Source: CAD feature listing. Evaluate the final solid. Frame: model axes, mm. A direction names the side the tool comes from. Round coordinates to 2 decimals unless told otherwise and drop trailing zeros. Loops run counter-clockwise (first coordinate to the right, second up) from the corner with the lowest first, then second, coordinate; pieces in that order, holes last. Notation, with made-up numbers: (62, 72) -> (71, 72) arc R31 ccw to (71, 111) -> close; hole circle Ø5 at (59, -21). An arc over 180 degrees is marked (long way). Put each result on its own line as item: value. Start each with the question number.
1. Material intervals for L1, parallel to Y at x = -5, z = 0; L2, parallel to Y at x = -9, z = -34; L3, parallel to Y at x = 22, z = -22.5, sorted ascending.
2. Cut plane A-A (x = -17). Return the cut outline in (y, z), then the cut area to 3 significant figures.
3. Cut plane B-B (y = -2). State how many separate pieces and enclosed holes the cut face has, then the cut area to 3 significant figures.
4. Set-up query: faces 4 (the flat face through (0, -22, 1)), 5 (the flat face through (17.426, 4, -1)), 6 (the flat face through (0, 5, 59)). Return all of +Z, -Z, +X, -X, +Y, -Y with unobstructed straight access to the full face (end or side cutting, diameter ignored); none if empty.
5. Contact query for flat-ended pins moving along their axis: pin 1 (1.2 mm diameter, centred on x = -24, z = -4, fed in from +Y); pin 2 (2 mm diameter, centred on x = 14.5, y = 9.5, fed in from +Z); pin 3 (8 mm diameter, centred on x = 26, y = -49, fed in from -Z). Output: stop coordinate, or through.
6. Draft query along Z for faces 1 (the cylindrical face through (-27.465, -19.214, 76.441)), 2 (the flat face through (-15, -5.34, 37)), 3 (the flat face through (30, -61, 24)). Return one class per face: pulls with the +Z half, pulls with the -Z half, needs draft (parallel to the pull), parting line crosses it, or undercut.
```python
from build123d import *
from build123d.topology import SkipClean

# Parameters (mm, degrees)
ESBO_O2_R                = 15
RESSALTO_EXTRUS_O1_DEPTH = 30
FILETE1_R                = 10
FILETE5_R                = 3
RESSALTO_EXTRUS_O3_DEPTH = 30
RESSALTO_EXTRUS_O4_START = -30
ESBO_O9_R                = 3
RESSALTO_EXTRUS_O4_DEPTH = 30
ESBO_O10_R               = 3
RESSALTO_EXTRUS_O5_DEPTH = 2
CORTE_EXTRUS_O1_START    = -0.3
ESBO_O14_R               = 3
CORTE_EXTRUS_O1_DEPTH    = 0.3
RESSALTO_EXTRUS_O6_START = -27
RESSALTO_EXTRUS_O6_DEPTH = 27


with BuildPart() as part:
    # Esboço1 → Revolução2 (revolve)
    with BuildSketch(Plane.XY, mode=Mode.PRIVATE) as revolu_o2_sk:
        Polygon((30, 69.858349347), (30, 4.858349347), (0, 4.858349347), (0, 19.858349347), (22.5, 19.858349347), (22.5, 69.858349347), (-30, 69.858349347), (-30, 85), (-25, 85), (-25, 79.858349347), (25, 79.858349347), (25, 84.858349347), (30, 84.858349347), align=None)
    revolve(revolu_o2_sk.sketch.rotate(Axis((-56.599013794, 4.858349347, 0), (1, 0, 0)), 90), axis=Axis((-56.599013794, 4.858349347, 0), (1, 0, 0)))

    # Esboço2 → Ressalto-extrusão1 (add)
    with BuildSketch(Plane(origin=(0, 0, 0), x_dir=(0, 0, -1), z_dir=(1, 0, 0))):
        with Locations(Location((0, 4.858349347, 0), (0, 0, 180))):
            Circle(ESBO_O2_R)
        with BuildLine():
            Line((-2.958039892, 5.358349347), (-4.5, 5.358349347))
            Line((-4.5, 5.358349347), (-4.5, 4.358349347))
            Line((-4.5, 4.358349347), (-2.958039892, 4.358349347))
            ThreePointArc((-2.958039892, 4.358349347), (-2.121320344, 2.737029004), (-0.5, 1.900309456))
            Line((-0.5, 1.900309456), (-0.5, 0.358349347))
            Line((-0.5, 0.358349347), (0.5, 0.358349347))
            Line((0.5, 0.358349347), (0.5, 1.900309456))
            ThreePointArc((0.5, 1.900309456), (2.121320344, 2.737029004), (2.958039892, 4.358349347))
            Line((2.958039892, 4.358349347), (4.5, 4.358349347))
            Line((4.5, 4.358349347), (4.5, 5.358349347))
            Line((4.5, 5.358349347), (2.958039892, 5.358349347))
            ThreePointArc((2.958039892, 5.358349347), (2.120440089, 6.98054958), (0.497545425, 7.81680309))
            Line((0.497545425, 7.81680309), (0.497545425, 9.358349347))
            Line((0.497545425, 9.358349347), (-0.5, 9.358349347))
            Line((-0.5, 9.358349347), (-0.5, 7.816389239))
            ThreePointArc((-0.5, 7.816389239), (-2.121320344, 6.979669691), (-2.958039892, 5.358349347))
        make_face(mode=Mode.SUBTRACT)
    extrude(amount=-RESSALTO_EXTRUS_O1_DEPTH)

    # Esboço4 → Revolução3 (revolve)
    with BuildSketch(Plane.XY, mode=Mode.PRIVATE) as revolu_o3_sk:
        Polygon((0, 59.226522002), (0, 4.858349347), (43.32899264, 4.858349347), (43.32899264, 74.582067629), align=None)
    revolve(revolu_o3_sk.sketch.rotate(Axis((-90.113441675, 4.858349347, 0), (1, 0, 0)), 270), axis=Axis((-90.113441675, 4.858349347, 0), (1, 0, 0)))

    # Esboço5 → Corte-Revolução3 (revolve, cut)
    with BuildSketch(Plane.XY, mode=Mode.PRIVATE) as corte_revolu_o3_sk:
        Polygon((43.32899264, 4.858349347), (43.32899264, 66.094541607), (32.672301871, 62.317871729), (22.015611102, 58.541201852), (17.426446921, 56.914828477), (17.426446921, 4.858349347), align=None)
    revolve(corte_revolu_o3_sk.sketch.rotate(Axis((17.426446921, 4.858349347, 0), (1, 0, 0)), 90), axis=Axis((17.426446921, 4.858349347, 0), (1, 0, 0)), mode=Mode.SUBTRACT)

    # Filete1
    filete1_edges = [part.edges().sort_by_distance(p)[0] for p in [
        (17.426446921, 4.858349347, -52.05647913),
    ]]
    fillet(filete1_edges, radius=FILETE1_R)

    # Filete5
    filete5_edges = [part.edges().sort_by_distance(p)[0] for p in [
        (30, 4.858349347, 65),
    ]]
    fillet(filete5_edges, radius=FILETE5_R)

    # Esboço7 → Ressalto-extrusão3 (add)
    with BuildSketch(Plane.ZY.offset(30)):
        with BuildLine():
            Line((-11, 15.056388374), (-64.195015383, 15.056388374))
            ThreePointArc((-64.195015383, 15.056388374), (-65, 4.858349347), (-64.195015383, -5.33968968))
            Line((-64.195015383, -5.33968968), (-11, -5.33968968))
            ThreePointArc((-11, -5.33968968), (-15, 4.858349347), (-11, 15.056388374))
        make_face()
        with BuildLine():
            Line((11, -5.33968968), (64.195015383, -5.33968968))
            ThreePointArc((64.195015383, -5.33968968), (65, 4.858349347), (64.195015383, 15.056388374))
            Line((64.195015383, 15.056388374), (11, 15.056388374))
            ThreePointArc((11, 15.056388374), (15, 4.858349347), (11, -5.33968968))
        make_face()
    extrude(amount=-RESSALTO_EXTRUS_O3_DEPTH)

    # Esboço9 → Ressalto-extrusão4 (add)
    with BuildSketch(Plane.ZY.offset(20.2).offset(RESSALTO_EXTRUS_O4_START)):
        with Locations((0, 4.858349347)):
            Circle(ESBO_O9_R)
    extrude(amount=RESSALTO_EXTRUS_O4_DEPTH)

    # Esboço10 → Ressalto-extrusão5 (add)
    with BuildSketch(Plane.ZY.offset(20.2)):
        with Locations((0, 4.858349347)):
            Circle(ESBO_O10_R)
    extrude(amount=RESSALTO_EXTRUS_O5_DEPTH)

    # Esboço14 → Corte-extrusão1 (cut)
    with SkipClean():  # the faces are left unmerged after this step: merging them gives an invalid solid
        with BuildSketch(Plane.ZY.offset(22.2).offset(CORTE_EXTRUS_O1_START)):
            with Locations((0, 4.858349347)):
                Circle(ESBO_O14_R)
        extrude(amount=CORTE_EXTRUS_O1_DEPTH, mode=Mode.SUBTRACT)
    add(part.part.scale(1), mode=Mode.REPLACE)  # the faces are merged on a copy

    # Esboço15 → Ressalto-extrusão6 (add)
    with SkipClean():  # the faces are left unmerged after this step: merging them gives an invalid solid
        with BuildSketch(Plane.ZY.offset(21.9).offset(RESSALTO_EXTRUS_O6_START)):
            with BuildLine():
                Line((-2.958039892, 5.358349347), (-4.5, 5.358349347))
                Line((-4.5, 5.358349347), (-4.5, 4.358349347))
                Line((-4.5, 4.358349347), (-2.958039892, 4.358349347))
                ThreePointArc((-2.958039892, 4.358349347), (-3, 4.858349347), (-2.958039892, 5.358349347))
            make_face()
            with BuildLine():
                Line((0.5, 7.816389239), (0.5, 9.358349347))
                Line((0.5, 9.358349347), (-0.497545425, 9.358349347))
                Line((-0.497545425, 9.358349347), (-0.497545425, 7.81680309))
                ThreePointArc((-0.497545425, 7.81680309), (0.00124461, 7.858349089), (0.5, 7.816389239))
            make_face()
            with BuildLine():
                Line((2.958039892, 4.358349347), (4.5, 4.358349347))
                Line((4.5, 4.358349347), (4.5, 5.358349347))
                Line((4.5, 5.358349347), (2.958039892, 5.358349347))
                ThreePointArc((2.958039892, 5.358349347), (3, 4.858349347), (2.958039892, 4.358349347))
            make_face()
            with BuildLine():
                ThreePointArc((2.958039892, 4.358349347), (3, 4.858349347), (2.958039892, 5.358349347))
                ThreePointArc((2.958039892, 5.358349347), (2.121320344, 6.979669691), (0.5, 7.816389239))
                ThreePointArc((0.5, 7.816389239), (0.00124461, 7.858349089), (-0.497545425, 7.81680309))
                ThreePointArc((-0.497545425, 7.81680309), (-2.120440089, 6.98054958), (-2.958039892, 5.358349347))
                ThreePointArc((-2.958039892, 5.358349347), (-3, 4.858349347), (-2.958039892, 4.358349347))
                ThreePointArc((-2.958039892, 4.358349347), (-2.121320344, 2.737029004), (-0.5, 1.900309456))
                ThreePointArc((-0.5, 1.900309456), (0, 1.858349347), (0.5, 1.900309456))
                ThreePointArc((0.5, 1.900309456), (2.121320344, 2.737029004), (2.958039892, 4.358349347))
            make_face()
            with BuildLine():
                Line((-0.5, 1.900309456), (-0.5, 0.358349347))
                Line((-0.5, 0.358349347), (0.5, 0.358349347))
                Line((0.5, 0.358349347), (0.5, 1.900309456))
                ThreePointArc((0.5, 1.900309456), (0, 1.858349347), (-0.5, 1.900309456))
            make_face()
        extrude(amount=RESSALTO_EXTRUS_O6_DEPTH)


solid = part.part
```
Solution:
1. L1: y = -70.14 to -60.14, -10.14 to 19.86, 69.86 to 79.86
1. L2: y = -61.99 to -50.54, -5.34 to 15.06, 60.26 to 71.71
1. L3: y = -66.69 to -56.12, -53.09 to -43.56, 53.28 to 62.81, 65.84 to 76.4
2. outline: circle Ø150 at (4.86, 0); hole (-5.34, -64.2) -> (-5.34, -11) arc R15 cw to (-5.34, 11) -> (-5.34, 64.2) arc R65 ccw to start; hole (15.06, -64.2) arc R65 ccw to (15.06, 64.2) -> (15.06, 11) arc R15 cw to (15.06, -11) -> close
2. area: 7,180 mm^2
3. separate pieces: 1
3. enclosed holes: 2
3. area: 7,660 mm^2
4. face 4: -X
4. face 5: +X
4. face 6: none
5. pin 1: stops at y = 79.78
5. pin 2: stops at z = 74.91
5. pin 3: stops at z = -62.56
6. face 1: parting line crosses it
6. face 2: undercut
6. face 3: needs draft
